from build123d import *

# Parameters (mm, degrees)
F0_R     = 2
F1_DEPTH = 6.35


# Not quite as in the source:
# - a length typed as a fraction of an inch, garbled in the dataset ("3 / 203.2 mm" for 3/8 in), is restored


with BuildPart() as f1:
    # F0 (on Front) → F1 (new body)
    with BuildSketch(Plane.XZ):
        Polygon((25, 45), (-18.65, 45), (-18.65, 38.65), (-25, 38.65), (-25, 30), (-25, -18.65), (-18.65, -18.65), (-18.65, -25), (18.65, -25), (18.65, -18.65), (25, -18.65), align=None)
        Circle(F0_R, mode=Mode.SUBTRACT)
        with Locations((0, 30)):
            Circle(F0_R, mode=Mode.SUBTRACT)
        with Locations((16, 30)):
            Circle(F0_R, mode=Mode.SUBTRACT)
    extrude(amount=F1_DEPTH)


solid = f1.part
Source: CAD feature listing. Evaluate the final solid. Frame: model axes, mm. A direction names the side the tool comes from. Give positions to 0.01 mm unless a question says otherwise; leave off trailing zeros. Write each loop counter-clockwise with the first axis right and the second up, starting at its lowest first coordinate (ties: lowest second). Pieces come first, ordered by that corner, then holes. Notation, with made-up numbers: (26.25, 18.5) -> (47.25, 18.5) arc R8 ccw to (47.25, 27.5) -> close; hole circle Ø10 at (-18.75, 78.25). An arc over 180 degrees is marked (long way). Write item = value, one per line.
Q1. Cut plane C-C on z = 30. Return loops of the section in (x, y), then the cut area to 3 significant figures.
Here are the results:
outline = (-25, -6.35) -> (-2, -6.35) -> (-2, 0) -> (-25, 0) -> close; (2, -6.35) -> (14, -6.35) -> (14, 0) -> (2, 0) -> close; (18, -6.35) -> (25, -6.35) -> (25, 0) -> (18, 0) -> close
area = 267 mm²
Q2. Mould query, pull axis X, two halves, no side actions, for faces 4 (the face through (0, -3, -2)), 5 (the face through (-22, -3, 38.65)), 6 (the face through (0, -3, 28)), 7 (the face through (-18.65, -3, 42)). Classes: +X half, -X half, draft (parallel to the pull), parting line (faces both ways), or undercut.
Here are the results:
face_4 = undercut
face_5 = draft
face_6 = undercut
face_7 = -X half
Q3. Line query: line 1 (Z direction, x = 0, y = -3.5); line 2 (Z direction, x = -21.5, y = -3); line 3 (Z direction, x = 21.5, y = -3.5). Output: solid intervals per line, ascending. Write a range as from..to.
Here are the results:
line_1 = -25..-2, 2..28, 32..45
line_2 = -18.65..38.65
line_3 = -18.65..45
Q4. Reachability of faces 1 (the face through (-22, -3, -18.65)), 2 (the face through (25, -3, 13)), 3 (the face through (22, -3, -18.65)) from +Z, -Z, +X, -X, +Y, -Y: full face, straight path, thin tool, end or side. Return the list, or none.
Here are the results:
face_1 = -Z, -X, +Y, -Y
face_2 = +Z, -Z, +X, +Y, -Y
face_3 = -Z, +X, +Y, -Y
Q5. First-contact query: pin 1 (4.5 mm diameter, centred on x = 16, z = 30, fed in from +Y); pin 2 (1.9 mm diameter, centred on y = -3, z = -23, fed in from +X); pin 3 (3 mm diameter, centred on x = -23, y = -3, fed in from -Z); pin 4 (3 mm diameter, centred on y = -4.5, z = 40.5, fed in from -X). Flat tips, straight axial feed; report the tip coordinate or a pass-through.
Here are the results:
pin_1 = 0
pin_2 = 18.65
pin_3 = -18.65
pin_4 = -18.65
Q6. Cut plane A-A on z = 0. Return loops of the section in (x, y), then the cut area to 3 significant figures.
Here are the results:
outline = (-25, -6.35) -> (-2, -6.35) -> (-2, 0) -> (-25, 0) -> close; (2, -6.35) -> (25, -6.35) -> (25, 0) -> (2, 0) -> close
area = 292 mm²
Q7. Cut plane D-D on x = 0. Return loops of the section in (y, z), then the cut area to 3 significant figures.
Here are the results:
outline = (-6.35, -25) -> (0, -25) -> (0, -2) -> (-6.35, -2) -> close; (-6.35, 2) -> (0, 2) -> (0, 28) -> (-6.35, 28) -> close; (-6.35, 32) -> (0, 32) -> (0, 45) -> (-6.35, 45) -> close
area = 394 mm²
Q8. Cut plane B-B on x = 16. Return loops of the section in (y, z).
Here are the results:
outline = (-6.35, -25) -> (0, -25) -> (0, 28) -> (-6.35, 28) -> close; (-6.35, 32) -> (0, 32) -> (0, 45) -> (-6.35, 45) -> close
